```python
from build123d import *

# Parameters (mm, degrees)
SKETCH1_R           = 1.5
BOSS_EXTRUDE1_DEPTH = 40
SKETCH1_3_R         = 1.5
CUT_EXTRUDE1_DEPTH  = 4
SKETCH3_R           = 11
SKETCH3_R_2         = 2.5
BOSS_EXTRUDE2_DEPTH = 2
SKETCH3_3_R         = 2.5
BOSS_EXTRUDE3_DEPTH = 23
CUT_EXTRUDE2_START  = -18
CUT_EXTRUDE2_DEPTH  = 18
CUT_EXTRUDE4_START  = -12
SKETCH5_W           = 55.059471924
SKETCH5_H           = 55.059471924
CUT_EXTRUDE4_DEPTH  = 20
SKETCH6_W           = 7.933477793
SKETCH6_H           = 18.223329292
BOSS_EXTRUDE4_DEPTH = 14
SKETCH7_W           = 3.936196897
SKETCH7_H           = 20.200423078
BOSS_EXTRUDE5_DEPTH = 7


with BuildPart() as part:
    # Sketch1 → Boss-Extrude1 (new body)
    # profile 1 of 5: a face of its own
    with BuildSketch(Plane(origin=(0, 0, 0), x_dir=(0, 0, -1), z_dir=(1, 0, 0))):
        Polygon((-15.65, 21.15), (0, 21.15), (15.65, 21.15), (21.15, 15.65), (21.15, 0), (21.15, -15.65), (15.65, -21.15), (0, -21.15), (-15.65, -21.15), (-21.15, -15.65), (-21.15, 0), (-21.15, 15.65), align=None)
        with Locations((-15.5, 15.5)):
            Circle(SKETCH1_R, mode=Mode.SUBTRACT)
        with Locations((-15.5, -15.5)):
            Circle(SKETCH1_R, mode=Mode.SUBTRACT)
        with Locations((15.5, -15.5)):
            Circle(SKETCH1_R, mode=Mode.SUBTRACT)
        with Locations((15.5, 15.5)):
            Circle(SKETCH1_R, mode=Mode.SUBTRACT)
    # profile 2 of 5: a face of its own
    with BuildSketch(Plane(origin=(0, 0, 0), x_dir=(0, 0, -1), z_dir=(1, 0, 0))):
        with Locations((15.5, -15.5)):
            Circle(SKETCH1_R)
    # profile 3 of 5: a face of its own
    with BuildSketch(Plane(origin=(0, 0, 0), x_dir=(0, 0, -1), z_dir=(1, 0, 0))):
        with Locations((-15.5, -15.5)):
            Circle(SKETCH1_R)
    # profile 4 of 5: a face of its own
    with BuildSketch(Plane(origin=(0, 0, 0), x_dir=(0, 0, -1), z_dir=(1, 0, 0))):
        with Locations((-15.5, 15.5)):
            Circle(SKETCH1_R)
    # profile 5 of 5: a face of its own
    with BuildSketch(Plane(origin=(0, 0, 0), x_dir=(0, 0, -1), z_dir=(1, 0, 0))):
        with Locations((15.5, 15.5)):
            Circle(SKETCH1_R)
    extrude(amount=BOSS_EXTRUDE1_DEPTH)

    # Sketch1<3> → Cut-Extrude1 (cut)
    with BuildSketch(Plane(origin=(0, 0, 0), x_dir=(0, 0, -1), z_dir=(1, 0, 0))):
        with Locations((-15.5, 15.5)):
            Circle(SKETCH1_3_R)
        with Locations((15.5, -15.5)):
            Circle(SKETCH1_3_R)
        with Locations((-15.5, -15.5)):
            Circle(SKETCH1_3_R)
        with Locations((15.5, 15.5)):
            Circle(SKETCH1_3_R)
    extrude(amount=CUT_EXTRUDE1_DEPTH, mode=Mode.SUBTRACT)

    # Sketch3 → Boss-Extrude2 (add)
    with BuildSketch(Plane.ZY):
        Circle(SKETCH3_R)
        Circle(SKETCH3_R_2, mode=Mode.SUBTRACT)
    extrude(amount=BOSS_EXTRUDE2_DEPTH)

    # Sketch3<3> → Boss-Extrude3 (add)
    with BuildSketch(Plane.ZY):
        Circle(SKETCH3_3_R)
    extrude(amount=BOSS_EXTRUDE3_DEPTH)

    # Sketch4 → Cut-Extrude2 (cut)
    with BuildSketch(Plane.ZY.offset(23).offset(CUT_EXTRUDE2_START)):
        with BuildLine():
            Line((-1.5, 2), (1.5, 2))
            ThreePointArc((1.5, 2), (0, 2.5), (-1.5, 2))
        make_face()
    extrude(amount=CUT_EXTRUDE2_DEPTH, mode=Mode.SUBTRACT)

    # Sketch5 → Cut-Extrude4 (cut)
    with BuildSketch(Plane(origin=(40, 0, 0), x_dir=(0, 0, -1), z_dir=(1, 0, 0)).offset(CUT_EXTRUDE4_START)):
        Rectangle(SKETCH5_W, SKETCH5_H)
        Polygon((-20.829250382, 14.625463373), (-14.625463373, 20.829250382), (14.625463373, 20.829250382), (20.829250382, 14.625463373), (20.829250382, -14.625463373), (14.625463373, -20.829250382), (-14.625463373, -20.829250382), (-20.829250382, -14.625463373), align=None, mode=Mode.SUBTRACT)
    extrude(amount=-CUT_EXTRUDE4_DEPTH, mode=Mode.SUBTRACT)

    # Sketch6 → Boss-Extrude4 (add)
    with BuildSketch(Plane.XZ.offset(21.15)):
        with Locations((31.966738897, 0)):
            Rectangle(SKETCH6_W, SKETCH6_H)
    extrude(amount=BOSS_EXTRUDE4_DEPTH)

    # Sketch7 → Boss-Extrude5 (add)
    with BuildSketch(Plane.XZ.offset(21.15)):
        with Locations((38.031901551, 0)):
            Rectangle(SKETCH7_W, SKETCH7_H)
    extrude(amount=BOSS_EXTRUDE5_DEPTH)


solid = part.part
```
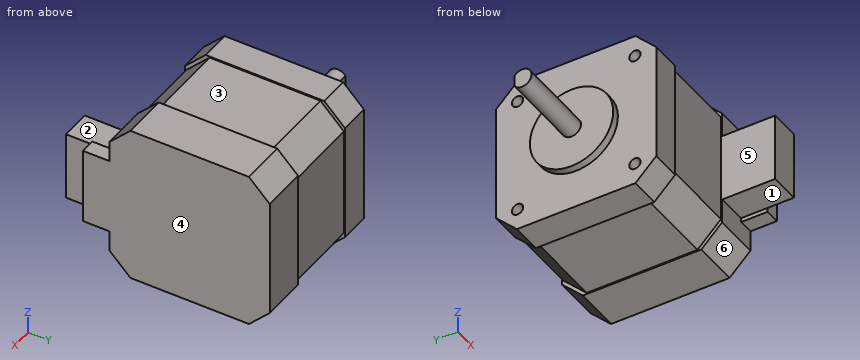
Check sheet for the modelled part. Datum: model origin and axes. Units: mm. Face numbers are marked on the shaded views. A direction names the side the tool comes from. Give positions to 0.01 mm unless a question says otherwise; leave off trailing zeros. Order: outer loops, then holes, each group sorted by start corner. A loop starts at its lowest first (then second) coordinate and runs counter-clockwise, first axis right, second up. Notation, with made-up numbers: M -37,5 L -17,5 A28 cw -17,27 Z; hole C 80,1 d4. An arc over 180 degrees is marked long. Answer in a Markdown table with one row per item. Add a question column.
Q1. Release check for a two-part mould opening along X. For the marked faces 4, 5 and 6 record: released by +X, released by -X, zero draft, split by the parting line, or undercut.
Q2. Gauge pin test, flat ends, axial feed: pin 1 Ø2 at (x, y) = (38, -25) entering from +Z; pin 2 Ø1.8 at (y, z) = (15.5, 15.5) entering from -X; pin 3 Ø1.2 at (x, y) = (38.5, -26) entering from -Z; pin 4 Ø2 at (x, z) = (-13, -5) entering from -Y. Record the tip position at first contact, or that the pin passes through.
Q3. Access from +Z, -Z, +X, -X, +Y, -Y to the whole of each face (thin tool, end or side, straight path). Record for the marked faces 1, 2 and 3.
Q4. Sectioned sample at C-C, the plane z = 0. Record the boundary of the cut face in (x, y), and give its area (3 significant figures).
Q5. Thickness scan on L1, parallel to Y at x = 0.9, z = -15.5; L2, parallel to Y at x = 2, z = -15. Record the ranges inside material, lowest first.
Q6. Sectioned sample at D-D, the plane y = 5. Record the boundary of the cut face in (x, z).
Q7. Sectioned sample at A-A, the plane z = 12. Record the boundary of the cut face in (x, y), and give its area (3 significant figures).
Verdict:
| question | item | result |
|---|---|---|
| 1 | face 4 | released by +X |
| 1 | face 5 | undercut |
| 1 | face 6 | zero draft |
| 2 | pin 1 | z = 10.1 |
| 2 | pin 2 | x = 4 |
| 2 | pin 3 | z = -10.1 |
| 2 | pin 4 | through |
| 3 | face 1 | -Z, -X, -Y |
| 3 | face 2 | +Z, -X, -Y |
| 3 | face 3 | +Z, +Y, -Y |
| 4 | outline | M -23,-2.5 L -2,-2.5 L -2,-11 L 0,-11 L 0,-21.15 L 8,-21.15 L 8,-20.83 L 28,-20.83 L 28,-35.15 L 35.93,-35.15 L 35.93,-21.15 L 36.06,-21.15 L 36.06,-28.15 L 40,-28.15 L 40,21.15 L 28,21.15 L 28,20.83 L 8,20.83 L 8,21.15 L 0,21.15 L 0,11 L -2,11 L -2,2.5 L -5,2.5 L -5,2 L -23,2 Z |
| 4 | area | 1,960 mm² |
| 5 | L1 | -21.15 to -17, -14 to 14, 17 to 21.15 |
| 5 | L2 | -21.15 to -16.91, -14.09 to 14.09, 16.91 to 21.15 |
| 6 | outline | M -2,-9.8 L 0,-9.8 L 0,-21.15 L 8,-21.15 L 8,-20.83 L 28,-20.83 L 28,-21.15 L 40,-21.15 L 40,21.15 L 28,21.15 L 28,20.83 L 8,20.83 L 8,21.15 L 0,21.15 L 0,9.8 L -2,9.8 Z |
| 7 | outline | M 0,-21.15 L 8,-21.15 L 8,-20.83 L 28,-20.83 L 28,-21.15 L 40,-21.15 L 40,21.15 L 28,21.15 L 28,20.83 L 8,20.83 L 8,21.15 L 0,21.15 Z |
| 7 | area | 1,680 mm² |
